For this review, take the finished solid that the model builds, in its own axes (mm). A direction names the side the tool comes from. Give positions to 0.01 mm unless a question says otherwise; leave off trailing zeros. Order: outer loops, then holes, each group sorted by start corner. A loop starts at its lowest first (then second) coordinate and runs counter-clockwise, first axis right, second up.
Item 1: For P1, Ø2.5, axis at x = 14.5, y = -16.5, coming from the -Z side (3 decimals); P2, Ø8, axis at x = -4, y = -18, coming from the +Z side (3 decimals); P3, Ø4.5, axis at x = -19.95, z = 26.16, coming from the -Y side; P4, Ø2.5, axis at x = -2, z = 27.5, coming from the -Y side, all flat-tipped, find the tip position at first contact; note any pin that passes through.
Item 2: Machinability: for faces 5 (the flat face through (32, -2.31, 0)), 6 (the flat face through (-1, -17, -10.088)), 7 (the flat face through (32, -13, 20.475)), 8 (the flat face through (0, -17, 22.475)), 9 (the flat face through (-32, -13, 20.475)), which of the approach directions +Z, -Z, +X, -X, +Y, -Y give a long, thin tool a straight path to every point of the face, cutting with its end or side? Answer none if there is none.
Item 3: Consider section A-A (z = -26.16). Give the boundary of the cut face in (x, y).
Item 4: For probe 1 along X at (y, z) = (-3.25, 26.16); probe 2 along Z at (x, y) = (-12, -16) (3 decimals); probe 3 along Z at (x, y) = (34, -17.75) (3 decimals), list the stretches that pass through material, from the lowest coordinate up.
Item 5: The part is to be moulded in two halves that separate along Y. For faces 1 (the cylindrical face through (-0.55, -21.97, 6.99)), 2 (the flat face through (0, -9.12, -27)), 3 (the cylindrical face through (19.83, -4.496, -23.413)), 4 (the flat face through (-1, -17, 10.088)), say which applies: released by +Y, released by -Y, zero draft, split by the parting line, or undercut.
Item 6: Consider section C-C (z = -5.5). Give the boundary of the cut face in (x, y).
Item 7: Consider section B-B (y = -11.5). Give the boundary of the cut face in (x, z) (3 decimals), plus the area to 3 significant figures.
Item 8: Consider section D-D (x = -6). Give the boundary of the cut face in (y, z) (1 decimal), plus the area to 3 significant figures.
```python
from build123d import *

# Parameters (mm, degrees)
RESSALTO_EXTRUS_O1_DEPTH = 25
ESBO_O2_R                = 2.75
CORTE_EXTRUS_O1_DEPTH    = 25
ESBO_O3_W                = 14.74
ESBO_O3_H                = 40.95
CORTE_EXTRUS_O2_DEPTH    = 2.31
CORTE_EXTRUS_O4_START    = -49.030903
ESBO_O7_W                = 9.03
ESBO_O7_H                = 15.88
CORTE_EXTRUS_O4_DEPTH    = 49.030903
CORTE_EXTRUS_O5_DEPTH    = 78.510903247


with BuildPart() as part:
    # Esboço1 → Ressalto-extrusão1 (new body)
    with BuildSketch(Plane(origin=(0, 0, 0), x_dir=(1, 0, 0), z_dir=(0, 1, 0))):
        Polygon((-24.515451624, -20.475), (-24.515451624, -31.505), (24.515451624, -31.505), (24.515451624, -20.475), (39.255451624, -20.475), (39.255451624, 20.475), (24.515451624, 20.475), (24.515451624, 31.505), (-24.515451624, 31.505), (-24.515451624, 20.475), (-39.255451624, 20.475), (-39.255451624, -20.475), align=None)
    extrude(amount=-RESSALTO_EXTRUS_O1_DEPTH)

    # Esboço2 → Corte-extrusão1 (cut)
    with BuildSketch(Plane(origin=(0, 0, 0), x_dir=(1, 0, 0), z_dir=(0, 1, 0))):
        with Locations(Location((-19.950451624, 26.16, 0), (0, 0, 270))):
            Circle(ESBO_O2_R)
        with Locations(Location((19.950451624, 26.16, 0), (0, 0, 90))):
            Circle(ESBO_O2_R)
        with Locations(Location((19.950451624, -26.16, 0), (0, 0, 270))):
            Circle(ESBO_O2_R)
        with Locations(Location((-19.950451624, -26.16, 0), (0, 0, 90))):
            Circle(ESBO_O2_R)
    extrude(amount=-CORTE_EXTRUS_O1_DEPTH, mode=Mode.SUBTRACT)

    # Esboço3 → Corte-extrusão2 (cut)
    with BuildSketch(Plane(origin=(0, 0, 0), x_dir=(1, 0, 0), z_dir=(0, 1, 0))):
        with Locations((31.885451624, 0)):
            Rectangle(ESBO_O3_W, ESBO_O3_H)
        with Locations((-31.885451624, 0)):
            Rectangle(ESBO_O3_W, ESBO_O3_H)
    extrude(amount=-CORTE_EXTRUS_O2_DEPTH, mode=Mode.SUBTRACT)

    # Esboço7 → Corte-extrusão4 (cut)
    with BuildSketch(Plane.ZY.offset(24.515451624).offset(CORTE_EXTRUS_O4_START)):
        with Locations((-26.99, -17.06)):
            Rectangle(ESBO_O7_W, ESBO_O7_H)
        with Locations((26.99, -17.06)):
            Rectangle(ESBO_O7_W, ESBO_O7_H)
    extrude(amount=CORTE_EXTRUS_O4_DEPTH, mode=Mode.SUBTRACT)

    # Esboço5 → Corte-extrusão5 (cut)
    with BuildSketch(Plane.ZY.offset(39.255451624)):
        with BuildLine():
            Line((-10.088028961, -25.000004947), (10.088017042, -25.000004947))
            ThreePointArc((10.088017042, -25.000004947), (6.988017042, -21.900004947), (10.088017042, -18.800004947))
            Line((10.088017042, -18.800004947), (10.088017042, -15.580004947))
            Line((10.088017042, -15.580004947), (9.685831834, -15.580004947))
            ThreePointArc((9.685831834, -15.580004947), (8.247865132, -15.007522497), (7.648994034, -13.580344232))
            Line((7.648994034, -13.580344232), (7.648994034, -13.080004947))
            Line((7.648994034, -13.080004947), (-7.649005954, -13.080004947))
            Line((-7.649005954, -13.080004947), (-7.649005954, -13.580344232))
            ThreePointArc((-7.649005954, -13.580344232), (-8.247877052, -15.007522497), (-9.685843753, -15.580004947))
            Line((-9.685843753, -15.580004947), (-10.088028961, -15.580004947))
            Line((-10.088028961, -15.580004947), (-10.088028961, -18.800004947))
            ThreePointArc((-10.088028961, -18.800004947), (-6.988028961, -21.900004947), (-10.088028961, -25.000004947))
        make_face()
    extrude(amount=-CORTE_EXTRUS_O5_DEPTH, mode=Mode.SUBTRACT)


solid = part.part
```
Resolved:
1. P1: stops at z = -22.475
1. P2: stops at z = 22.475
1. P3: passes through
1. P4: stops at y = -9.12
2. face 5: +Z, -Z, +X, +Y
2. face 6: +X, -X
2. face 7: +Z, +X, +Y, -Y
2. face 8: +Z, +X, -X, -Y
2. face 9: +Z, -X, +Y, -Y
3. outline: (-24.52, -9.12) - (-22.7, -9.12) - (-22.7, 0) - (-24.52, 0) - close; (-17.2, -9.12) - (17.2, -9.12) - (17.2, 0) - (-17.2, 0) - close; (22.7, -9.12) - (24.52, -9.12) - (24.52, 0) - (22.7, 0) - close
4. probe 1: x = -24.52 to -22.7, -17.2 to 17.2, 22.7 to 24.52
4. probe 2: z = -22.475 to -10.088, 10.088 to 22.475
4. probe 3: z = -20.475 to -10.088, 10.088 to 20.475
5. face 1: undercut
5. face 2: released by -Y
5. face 3: zero draft
5. face 4: undercut
6. outline: (-39.26, -13.08) - (39.26, -13.08) - (39.26, -2.31) - (24.52, -2.31) - (24.52, 0) - (-24.52, 0) - (-24.52, -2.31) - (-39.26, -2.31) - close
7. outline: (-39.255, -20.475) - (-24.515, -20.475) - (-24.515, -22.475) - (24.515, -22.475) - (24.515, -20.475) - (39.255, -20.475) - (39.255, 20.475) - (24.515, 20.475) - (24.515, 22.475) - (-24.515, 22.475) - (-24.515, 20.475) - (-39.255, 20.475) - close
7. area: 3,410 mm2
8. outline: (-25, -22.5) - (-9.1, -22.5) - (-9.1, -31.5) - (0, -31.5) - (0, 31.5) - (-9.1, 31.5) - (-9.1, 22.5) - (-25, 22.5) - (-25, 10.1) arc R3.1 ccw to (-18.8, 10.1) - (-15.6, 10.1) - (-15.6, 9.7) arc R2 ccw to (-13.6, 7.6) - (-13.1, 7.6) - (-13.1, -7.6) - (-13.6, -7.6) arc R2 ccw to (-15.6, -9.7) - (-15.6, -10.1) - (-18.8, -10.1) arc R3.1 ccw to (-25, -10.1) - close
8. area: 1,090 mm2
